from build123d import *

# Parameters (mm, degrees)
SKETCH2_R           = 4.7
SKETCH2_R_2         = 3
BOSS_EXTRUDE1_DEPTH = 3.7
SKETCH3_R           = 3
CUT_EXTRUDE1_DEPTH  = 19.753399692
FILLET1_R           = 0.5
FILLET2_R           = 0.3


with BuildPart() as part:
    # Sketch1 → Revolve1 (revolve)
    with BuildSketch(Plane(origin=(0, 0, 0), x_dir=(0, 0, -1), z_dir=(1, 0, 0))):
        Polygon((-13, -2.35), (-13, -1.883523848), (-10.110793586, -0.15), (-10.110793586, 0.65), (-13, 2.383523848), (-13, 2.85), (-10, 1.05), (0, 1.05), (0, -0.55), (-10, -0.55), align=None)
    revolve(axis=Axis((0, 0, 0), (0, -1, 0)))

    # Sketch2 → Boss-Extrude1 (add)
    with BuildSketch(Plane(origin=(0, 1.05, 0), x_dir=(1, 0, 0), z_dir=(0, 1, 0))):
        with Locations(Location((0, 0, 0), (0, 0, 270))):
            Circle(SKETCH2_R)
        with Locations(Location((0, 0, 0), (0, 0, 270))):
            Circle(SKETCH2_R_2, mode=Mode.SUBTRACT)
    boss_extrude1 = extrude(amount=BOSS_EXTRUDE1_DEPTH)

    # Sketch3 → Cut-Extrude1 (cut, through all)
    with BuildSketch(Plane(origin=(0, 1.05, 0), x_dir=(1, 0, 0), z_dir=(0, 1, 0))):
        with Locations(Location((0, 0, 0), (0, 0, 90))):
            Circle(SKETCH3_R)
    extrude(amount=-CUT_EXTRUDE1_DEPTH, mode=Mode.SUBTRACT)

    # Mirror1: Boss-Extrude1 across plane
    add(boss_extrude1.mirror(Plane.ZX.offset(0.25)))

    # Fillet1
    fillet1_edges = [part.edges().sort_by_distance(p)[0] for p in [
        (0, 4.75, -4.7),
        (0, -4.25, -4.7),
    ]]
    fillet(fillet1_edges, radius=FILLET1_R)

    # Fillet2
    fillet2_edges = [part.edges().sort_by_distance(p)[0] for p in [
        (0, 1.05, -4.7),
        (0, -0.55, -4.7),
        (0, 1.05, -10),
        (0, -0.55, -10),
    ]]
    fillet(fillet2_edges, radius=FILLET2_R)


solid = part.part
Design review of the part built by this model. Coordinates are the model's own, in mm. A direction names the side the tool comes from. Coordinates: 2 decimals unless noted, no trailing zeros. Order: outer loops, then holes, each group sorted by start corner. A loop starts at its lowest first (then second) coordinate and runs counter-clockwise, first axis right, second up. Notation, with made-up numbers: (79, -25.5) -> (99, -25.5) arc R36 cw to (99, 9.5) -> close; hole circle Ø6 at (44.25, 58). An arc over 180 degrees is marked (long way). One line per item, written item: value.
1) To check wall thickness, follow probe 1 along X at (y, z) = (1.5, 2.25); probe 2 along X at (y, z) = (2.2, 0); probe 3 along X at (y, z) = (-3.45, 0). State the ranges of each line that lie inside material, in increasing order. Write a range as [from, to].
Output values:
probe 1: x = [-11.31, -10.51], [-4.13, -1.98], [1.98, 4.13], [10.51, 11.31]
probe 2: x = [-12.69, -11.92], [-4.7, -3], [3, 4.7], [11.92, 12.69]
probe 3: x = [-4.7, -3], [3, 4.7]
2) Clearance check with flat-ended pins moving along their axes: P1, Ø3, axis at x = -5, y = -0.5, coming from the -Z side; P2, Ø1, axis at x = 7.5, z = 1.5, coming from the -Y side; P3, Ø5, axis at x = -3.5, y = 1, coming from the +Z side; P4, Ø5, axis at x = 0, z = 0, coming from the +Y side. State where each tip first meets the part, or that it passes through.
Output values:
P1: stops at z = -12.23
P2: stops at y = -0.55
P3: stops at z = 12.92
P4: passes through
3) Draft analysis for pull direction Y (two halves, no side actions). For faces 6 (the face through (3, -4.25, -1)), 7 (the face through (7.91, -2.113, -10.316)), 8 (the face through (6.152, 0.256, -8.024)), state which applies: +Y half, -Y half, draft (parallel to the pull), parting line (faces both ways), or undercut.
Output values:
face 6: -Y half
face 7: draft
face 8: undercut
4) We need section A-A, the plane y = 3.5. Give the boundary of the cut face in (x, z).
Output values:
outline: circle Ø9.4 at (0, 0); hole circle Ø6 at (0, 0)
5) Machinability: for faces 1 (the face through (10.007, -0.234, -2.222)), 2 (the face through (3, 4.75, -1)), 3 (the face through (1.412, -2.28, 4.483)), 4 (the face through (1.412, 2.78, 4.483)), 5 (the face through (7.91, 2.62, -10.316)), which of the approach directions +Z, -Z, +X, -X, +Y, -Y give a long, thin tool a straight path to every point of the face, cutting with its end or side? Answer none if there is none.
Output values:
face 1: none
face 2: +Z, -Z, +X, -X, +Y
face 3: -Y
face 4: +Y
face 5: +Y, -Y
